Build history of the part. All positions in model axes, mm. Face numbers are marked on the shaded views. A direction names the side the tool comes from. Round coordinates to 2 decimals unless told otherwise and drop trailing zeros. Loops run counter-clockwise (first coordinate to the right, second up) from the corner with the lowest first, then second, coordinate; pieces in that order, holes last. Notation, with made-up numbers: (-32, 64) - (13, 64) arc R28 ccw to (13, 99) - close; hole circle Ø7 at (7.25, -5). An arc over 180 degrees is marked (long way). One line per question, with ' | ' between items. Start each with the question number.
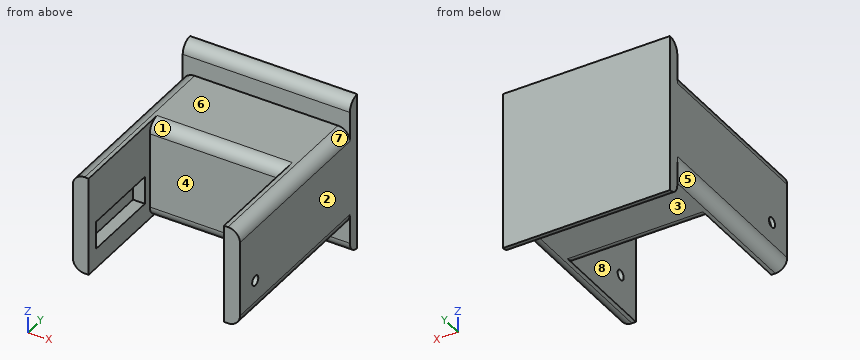
from build123d import *

# Parameters (mm, degrees)
F0_W     = 42
F0_H     = 40
F1_DEPTH = 3
F2_W     = 42
F2_H     = 25
F3_DEPTH = 45
F4_W     = 34
F4_H     = 25
F5_DEPTH = 32.501
F6_W     = 20
F6_H     = 7
F7_DEPTH = 3
F8_R     = 1.25
F9_DEPTH = 42.001
F10_R    = 2.99999


# Not quite as in the source:
# - a fillet or chamfer is up to 0.001 mm smaller than in the source, because OpenCascade refuses the exact size


with BuildPart() as f1:
    # F0 (on Front) → F1 (new body)
    with BuildSketch(Plane.XZ):
        with Locations((-2.4715067595, 12.8215752275)):
            Rectangle(F0_W, F0_H)
    extrude(amount=F1_DEPTH)

    # F2 (on face) → F3 (join)
    with BuildSketch(Plane.XZ.offset(3)):
        with Locations((-2.4715067595, 12.8215752275)):
            Rectangle(F2_W, F2_H)
    extrude(amount=F3_DEPTH)

    # F4 (on face) → F5 (cut, through all)
    with BuildSketch(Plane(origin=(0, 0, 0.3215752275), x_dir=(1, 0, 0), z_dir=(0, 0, -1))):
        with Locations((-2.4715067595, 35.5)):
            Rectangle(F4_W, F4_H)
    extrude(amount=-F5_DEPTH, mode=Mode.SUBTRACT)

    # F6 (on face) → F7 (cut)
    with BuildSketch(Plane.YZ.offset(-19.4715067595)):
        with Locations((-35, 8.8215752275)):
            Rectangle(F6_W, F6_H)
    extrude(amount=-F7_DEPTH, mode=Mode.SUBTRACT)

    # F8 (on face) → F9 (cut, through all)
    with BuildSketch(Plane(origin=(-23.4715067595, 0, 0), x_dir=(0, -1, 0), z_dir=(-1, 0, 0))):
        with Locations((41.75, 8.8215752275)):
            Circle(F8_R)
    extrude(amount=-F9_DEPTH, mode=Mode.SUBTRACT)

    # F10 (radius 3 in the source; OpenCascade refuses exactly that, so slightly less here)
    f10_edges = [f1.edges().sort_by_distance(p)[0] for p in [
        (-23.471507, -25.5, 0.321575),
        (18.528493, -25.5, 0.321575),
        (-23.471507, -25.5, 25.321575),
        (18.528493, -25.5, 25.321575),
        (-2.471507, -23, 25.321575),
        (-2.471507, -23, 0.321575),
        (-2.471507, -3, -7.178425),
        (-2.471507, -3, 32.821575),
    ]]
    fillet(f10_edges, radius=F10_R)


solid = f1.part
1) Saw through at A-A on y = -41.75. Write the cut outline in (x, z).
2) Two-plate mould, pull along X, no slides. Class the marked faces 6, 7 and 8: +X half, -X half, draft (parallel to the pull), parting line (faces both ways), or undercut.
3) Saw through at C-C on y = -13.5. Write the cut outline in (x, z), and give its area (3 significant figures).
4) Wall check: line 1 (Y direction, x = -13.5, z = 5.5); line 2 (Z direction, x = -22.95, y = -41.75); line 3 (Y direction, x = 8.5, z = 26). Give the ranges that are in metal, low to high. Write a range as [from, to].
5) Saw through at B-B on z = 13. Write the cut outline in (x, y), and give its area (3 significant figures).
6) Drop flat-ended pins along their axis: pin 1 (1.5 mm diameter, centred on y = -41.75, z = 8.82, fed in from +X) (3 decimals); pin 2 (10 mm diameter, centred on x = 13, y = -26.5, fed in from -Z); pin 3 (2 mm diameter, centred on x = -3, z = -1, fed in from -Y); pin 4 (5.5 mm diameter, centred on x = -0.5, z = 15, fed in from -Y). Give the stop position or say it passes through.
7) Tool access for the marked faces 1, 2, 3, 4 and 5: list every direction of +Z, -Z, +X, -X, +Y, -Y with a clear straight run to the whole face (end or side of a thin tool).
Answer key:
1) outline: (-23.47, 3.32) arc R3 ccw to (-20.47, 0.32) - (-19.47, 0.32) - (-19.47, 5.32) - (-22.47, 5.32) - (-22.47, 7.57) - (-23.47, 7.57) - close; (-23.47, 10.07) - (-22.47, 10.07) - (-22.47, 12.32) - (-19.47, 12.32) - (-19.47, 25.32) - (-20.47, 25.32) arc R3 ccw to (-23.47, 22.32) - close; (14.53, 0.32) - (15.53, 0.32) arc R3 ccw to (18.53, 3.32) - (18.53, 7.57) - (14.53, 7.57) - close; (14.53, 10.07) - (18.53, 10.07) - (18.53, 22.32) arc R3 ccw to (15.53, 25.32) - (14.53, 25.32) - close
2) face 6: draft | face 7: +X half | face 8: undercut
3) outline: (-23.47, 3.32) arc R3 ccw to (-20.47, 0.32) - (15.53, 0.32) arc R3 ccw to (18.53, 3.32) - (18.53, 22.32) arc R3 ccw to (15.53, 25.32) - (-20.47, 25.32) arc R3 ccw to (-23.47, 22.32) - close | area: 1,040 mm²
4) line 1: [-23, 0] | line 2: [1.63, 7.57], [10.07, 24.01] | line 3: [-3, 0]
5) outline: (-23.47, -48) - (-19.47, -48) - (-19.47, -23) - (14.53, -23) - (14.53, -48) - (18.53, -48) - (18.53, 0) - (-23.47, 0) - close | area: 1,170 mm²
6) pin 1: through | pin 2: z = 0.32 | pin 3: y = -3 | pin 4: y = -23
7) face 1: +Z, -Y | face 2: +Z, -Z, +X, +Y, -Y | face 3: -Z, +X, -X, -Y | face 4: +Z, -Z, -Y | face 5: -Z, -X, -Y
